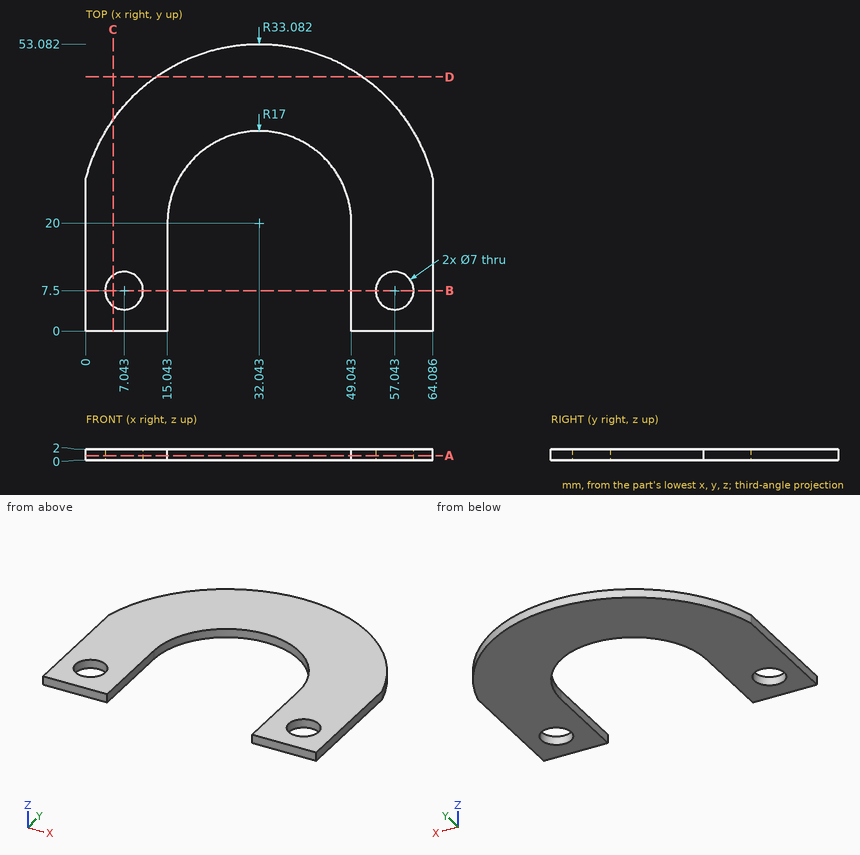
Print and shaded views of the part. All mm, measured from the part's lowest x, y and z. Round coordinates to 2 decimals unless told otherwise and drop trailing zeros. Order: outer loops, then holes, each group sorted by start corner. A loop starts at its lowest first (then second) coordinate and runs counter-clockwise, first axis right, second up.
Q1. Slice it at D-D (y = 47). Write the cut outline in (x, z).
Q2. Wall check: L1, parallel to X at y = 18, z = 0.95 (1 decimal); L2, parallel to Y at x = 7.5, z = 0.95 (1 decimal); L3, parallel to Y at x = 5, z = 1.25 (1 decimal). Give the ranges that are in metal, low to high.
Q3. Drop flat-ended pins along their axis: pin 1 (1 mm diameter, centred on x = 7.5, y = 39.5, fed in from -Z); pin 2 (5.5 mm diameter, centred on x = 57.04, y = 7.5, fed in from +Z). Give the stop position or say it passes through.
Q4. Slice it at C-C (x = 5). Write the cut outline in (y, z) (1 decimal).
Q5. Slice it at A-A (z = 0.8). Write the cut outline in (x, y) (1 decimal).
Q6. Slice it at B-B (y = 7.5). Write the cut outline in (x, z) (1 decimal).
Results below:
1. outline: (12.93, 0) - (51.16, 0) - (51.16, 2) - (12.93, 2) - close
2. L1: x = 0 to 15, 49 to 64.1
2. L2: y = 0 to 4, 11 to 42.2
2. L3: y = 0 to 4.7, 10.3 to 39.1
3. pin 1: stops at z = 0
3. pin 2: passes through
4. outline: (0, 0) - (4.7, 0) - (4.7, 2) - (0, 2) - close; (10.3, 0) - (39.1, 0) - (39.1, 2) - (10.3, 2) - close
5. outline: (0, 0) - (15, 0) - (15, 20) arc R17 cw to (49, 20) - (49, 0) - (64.1, 0) - (64.1, 28.2) arc R33.1 ccw to (0, 28.2) - close; hole circle Ø7 at (7, 7.5); hole circle Ø7 at (57, 7.5)
6. outline: (0, 0) - (3.5, 0) - (3.5, 2) - (0, 2) - close; (10.5, 0) - (15, 0) - (15, 2) - (10.5, 2) - close; (49, 0) - (53.5, 0) - (53.5, 2) - (49, 2) - close; (60.5, 0) - (64.1, 0) - (64.1, 2) - (60.5, 2) - close
